```python
from build123d import *

# Parameters (mm, degrees)
SKETCH1_R           = 13
SKETCH1_R_2         = 11.25
BOSS_EXTRUDE1_DEPTH = 1.2
SKETCH2_R           = 13
SKETCH2_R_2         = 11.75
BOSS_EXTRUDE2_DEPTH = 50
CHAMFER1_SIZE       = 0.5
BOSS_EXTRUDE3_DEPTH = 75
SKETCH4_W           = 52
SKETCH4_H           = 24
BOSS_EXTRUDE4_DEPTH = 26
SKETCH5_W           = 24
SKETCH5_H           = 24
BOSS_EXTRUDE5_DEPTH = 5
CUT_EXTRUDE1_DEPTH  = 112.130553854
FILLET1_R           = 10


with BuildPart() as part:
    # Sketch1 → Boss-Extrude1 (new body)
    with BuildSketch(Plane(origin=(0, 0, 0), x_dir=(1, 0, 0), z_dir=(0, 1, 0))):
        with Locations(Location((0, 0, 0), (0, 0, 270))):
            Circle(SKETCH1_R)
        with Locations(Location((0, 0, 0), (0, 0, 270))):
            Circle(SKETCH1_R_2, mode=Mode.SUBTRACT)
    extrude(amount=BOSS_EXTRUDE1_DEPTH)

    # Sketch2 → Boss-Extrude2 (add)
    with BuildSketch(Plane(origin=(0, 1.2, 0), x_dir=(1, 0, 0), z_dir=(0, 1, 0))):
        with Locations(Location((0, 0, 0), (0, 0, 270))):
            Circle(SKETCH2_R)
        with Locations(Location((0, 0, 0), (0, 0, 270))):
            Circle(SKETCH2_R_2, mode=Mode.SUBTRACT)
    extrude(amount=BOSS_EXTRUDE2_DEPTH)

    # Chamfer1
    chamfer1_edges = [part.edges().sort_by_distance(p)[0] for p in [
        (0, 1.2, -11.25),
    ]]
    chamfer(chamfer1_edges, length=CHAMFER1_SIZE - 0.0001)  # a hair under: the kernel refuses the full size

    # Sketch3 → Boss-Extrude3 (add)
    with BuildSketch(Plane.XZ):
        with BuildLine():
            Line((-13, 0), (-13, 13))
            Line((-13, 13), (0, 13))
            Line((0, 13), (13, 13))
            Line((13, 13), (13, 0))
            Line((13, 0), (11.75, 0))
            ThreePointArc((11.75, 0), (0, 11.75), (-11.75, 0))
            Line((-11.75, 0), (-13, 0))
        make_face()
    extrude(amount=-BOSS_EXTRUDE3_DEPTH)

    # Sketch4 → Boss-Extrude4 (add)
    with BuildSketch(Plane(origin=(13, 0, 0), x_dir=(0, 0, -1), z_dir=(1, 0, 0))):
        with Locations((-39, 63)):
            Rectangle(SKETCH4_W, SKETCH4_H)
    extrude(amount=-BOSS_EXTRUDE4_DEPTH)

    # Sketch5 → Boss-Extrude5 (add)
    # profile 1 of 2: a face of its own
    with BuildSketch(Plane.XY.offset(65)):
        with Locations((-25, 63)):
            Rectangle(SKETCH5_W, SKETCH5_H)
        Polygon((-27.828427125, 63), (-25, 65.828427125), (-22.171572875, 63), (-25, 60.171572875), align=None, mode=Mode.SUBTRACT)
    # profile 2 of 2: a face of its own
    with BuildSketch(Plane.XY.offset(65)):
        with Locations((25, 63)):
            Rectangle(SKETCH5_W, SKETCH5_H)
        Polygon((22.171572875, 63), (25, 65.828427125), (27.828427125, 63), (25, 60.171572875), align=None, mode=Mode.SUBTRACT)
    extrude(amount=-BOSS_EXTRUDE5_DEPTH)

    # Sketch6 → Cut-Extrude1 (cut, through all)
    with BuildSketch(Plane.ZY.offset(13)):
        Polygon((0, 51.2), (-13, 38.2), (-13, 51.2), align=None)
    extrude(amount=-CUT_EXTRUDE1_DEPTH, mode=Mode.SUBTRACT)

    # Fillet1
    fillet1_edges = [part.edges().sort_by_distance(p)[0] for p in [
        (-12.375, 75, 0),
        (12.375, 75, 0),
    ]]
    fillet(fillet1_edges, radius=FILLET1_R)


solid = part.part
```
Can you work these out from the model? Positions are in its coordinate system, mm. A direction names the side the tool comes from. Coordinates: 2 decimals unless noted, no trailing zeros. Order: outer loops, then holes, each group sorted by start corner. A loop starts at its lowest first (then second) coordinate and runs counter-clockwise, first axis right, second up. Notation, with made-up numbers: (73, 6.25) - (119, 6.25) arc R15 ccw to (119, 27.25) - close; hole circle Ø10 at (64.25, 73.25). An arc over 180 degrees is marked (long way). Answer in a Markdown table with one row per item.
1. For faces 5 (the flat face through (22, 63, 60)), 6 (the flat face through (-26.394, 61.566, 62.535)), 7 (the flat face through (-2, 39.4, -11.8)), 8 (the flat face through (-13, 55, 24)), which set-ups out of +Z, -Z, +X, -X, +Y, -Y let a thin tool reach every point of the face, with its end or its side?
Reply:
| item | result |
|---|---|
| face 5 | -Z, +X, +Y, -Y |
| face 6 | +Z, -Z |
| face 7 | -Z, +X, -X, +Y |
| face 8 | -Z, -X, +Y, -Y |
2. For pin 1 (19 mm diameter, centred on x = 23.5, y = 68.5, fed in from -Z); pin 2 (12 mm diameter, centred on y = 14, z = 18, fed in from +X); pin 3 (0.6 mm diameter, centred on x = -12, y = 58.5, fed in from -Z); pin 4 (5 mm diameter, centred on x = -11.5, z = -4.5, fed in from -Y), each with a flat end and sliding along its axis, tell me the tip position at first contact or that it passes through.
Reply:
| item | result |
|---|---|
| pin 1 | stops at z = 60 |
| pin 2 | stops at x = 13 |
| pin 3 | stops at z = 0 |
| pin 4 | stops at y = 0 |
3. If I drill on line 1 along X through (y, z) = (0.1, 0); line 2 along Z through (x, y) = (-0.5, 9); line 3 along Z through (x, y) = (22, 60), over which ranges is the centre line in solid material (lowest first)?
Reply:
| item | result |
|---|---|
| line 1 | x = -13 to -11.25, 11.25 to 13 |
| line 2 | z = -12.99 to -11.74, 11.74 to 13 |
| line 3 | z = 60 to 65 |
4. Suppose I cut it at B-B (y = 44.5). Please give me the cut outline in (x, z).
Reply:
| item | result |
|---|---|
| outline | (-13, 0) arc R13 ccw to (-11.14, -6.7) - (-9.65, -6.7) arc R11.75 cw (long way) to (9.65, -6.7) - (11.14, -6.7) arc R13 ccw to (13, 0) - (13, 13) - (-13, 13) - close |
5. Suppose I cut it at D-D (z = 32). Please give me the cut outline in (x, y), and give its area (3 significant figures).
Reply:
| item | result |
|---|---|
| outline | (-13, 51) - (13, 51) - (13, 75) - (-13, 75) - close |
| area | 624 mm^2 |
6. Suppose I cut it at C-C (x = -18.5). Please give me the cut outline in (y, z), and give its area (3 significant figures).
Reply:
| item | result |
|---|---|
| outline | (51, 60) - (75, 60) - (75, 65) - (51, 65) - close |
| area | 120 mm^2 |
7. Suppose I cut it at A-A (y = 25). Please give me the cut outline in (x, z).
Reply:
| item | result |
|---|---|
| outline | (-13, 0) arc R13 ccw to (13, 0) - (13, 13) - (-13, 13) - close; hole circle Ø23.5 at (0, 0) |
8. If we mould it in two halves opening along X, with no side actions, what happens to faces 1 (the flat face through (-28, 63, 60)), 2 (the flat face through (-23.566, 61.606, 62.535)), 3 (the flat face through (13, 55, 24)), 4 (the flat face through (23.566, 64.394, 62.535))? For each: pulls with the +X half, pulls with the -X half, needs draft (parallel to the pull), parting line crosses it, or undercut.
Reply:
| item | result |
|---|---|
| face 1 | needs draft |
| face 2 | undercut |
| face 3 | pulls with the +X half |
| face 4 | undercut |
